The drawing under review shows one solid part. Ordinate dimensions are in mm from its lowest x, y, z. A direction names the side the tool comes from. Give positions to 0.01 mm unless a question says otherwise; leave off trailing zeros. Order: outer loops, then holes, each group sorted by start corner. A loop starts at its lowest first (then second) coordinate and runs counter-clockwise, first axis right, second up. Notation, with made-up numbers: (53.25, 34.5) - (96.25, 34.5) arc R27 ccw to (96.25, 51.5) - close; hole circle Ø8 at (2.5, 31). An arc over 180 degrees is marked (long way). Use CSV: the item, a comma, the result in double quotes.
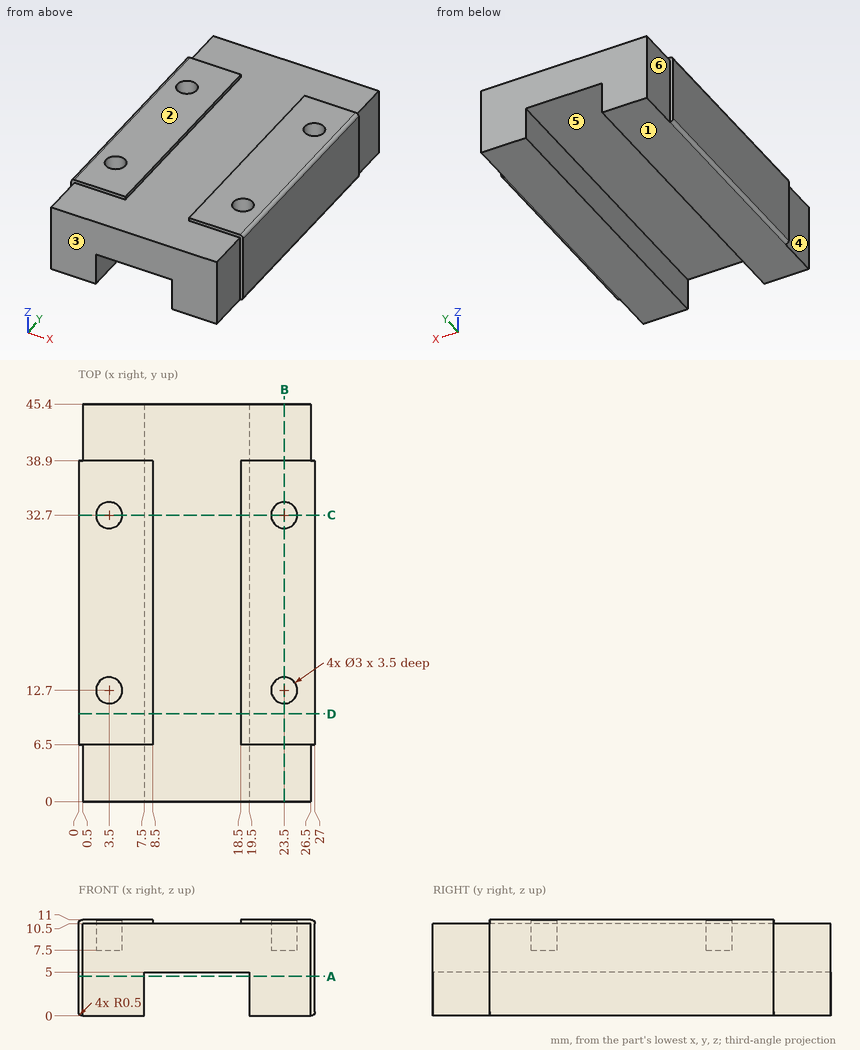
Item 1: Take a section at B-B, the plane x = 23.5. Give the boundary of the cut face in (y, z).
Results list:
outline,"(0, 0) - (45.4, 0) - (45.4, 10.5) - (38.9, 10.5) - (38.9, 11) - (34.2, 11) - (34.2, 7.5) - (31.2, 7.5) - (31.2, 11) - (14.2, 11) - (14.2, 7.5) - (11.2, 7.5) - (11.2, 11) - (6.5, 11) - (6.5, 10.5) - (0, 10.5) - close"
Item 2: Take a section at A-A, the plane z = 4.5. Give the boundary of the cut face in (x, y).
Results list:
outline,"(0, 6.5) - (0.5, 6.5) - (0.5, 0) - (7.5, 0) - (7.5, 45.4) - (0.5, 45.4) - (0.5, 38.9) - (0, 38.9) - close; (19.5, 0) - (26.5, 0) - (26.5, 6.5) - (27, 6.5) - (27, 38.9) - (26.5, 38.9) - (26.5, 45.4) - (19.5, 45.4) - close"
Item 3: Take a section at D-D, the plane y = 10. Give the boundary of the cut face in (x, z).
Results list:
outline,"(0, 0.5) arc R0.5 ccw to (0.5, 0) - (7.5, 0) - (7.5, 5) - (19.5, 5) - (19.5, 0) - (26.5, 0) arc R0.5 ccw to (27, 0.5) - (27, 10.5) arc R0.5 ccw to (26.5, 11) - (18.5, 11) - (18.5, 10.5) - (8.5, 10.5) - (8.5, 11) - (0.5, 11) arc R0.5 ccw to (0, 10.5) - close"
Item 4: Take a section at C-C, the plane y = 32.7. Give the boundary of the cut face in (x, z).
Results list:
outline,"(0, 0.5) arc R0.5 ccw to (0.5, 0) - (7.5, 0) - (7.5, 5) - (19.5, 5) - (19.5, 0) - (26.5, 0) arc R0.5 ccw to (27, 0.5) - (27, 10.5) arc R0.5 ccw to (26.5, 11) - (25, 11) - (25, 7.5) - (22, 7.5) - (22, 11) - (18.5, 11) - (18.5, 10.5) - (8.5, 10.5) - (8.5, 11) - (5, 11) - (5, 7.5) - (2, 7.5) - (2, 11) - (0.5, 11) arc R0.5 ccw to (0, 10.5) - close"
Item 5: Tool access review of the marked faces 4, 5 and 6: name each direction out of +Z, -Z, +X, -X, +Y, -Y from which nothing blocks a thin tool from reaching the whole face with its end or side.
Results list:
face 4,"+Z, -Z, -X, -Y"
face 5,"-Z, +Y, -Y"
face 6,"+Z, -Z, -X, +Y"
Item 6: Wall thickness on L1, parallel to X at y = 12.7, z = 8.9; L2, parallel to Y at x = 3.5, z = 9.15; L3, parallel to X at y = 25.5, z = 3.5: over which ranges is each line inside the solid? List them lowest first.
Results list:
L1,"x = 0 to 2, 5 to 22, 25 to 27"
L2,"y = 0 to 11.2, 14.2 to 31.2, 34.2 to 45.4"
L3,"x = 0 to 7.5, 19.5 to 27"
Item 7: Mouldability with a two-part tool opening along Z and no side actions: class the marked faces 1, 2 and 3 as pulls with the +Z half, pulls with the -Z half, needs draft (parallel to the pull), parting line crosses it, or undercut.
Results list:
face 1,"pulls with the -Z half"
face 2,"pulls with the +Z half"
face 3,"needs draft"
Item 8: Clearance check with flat-ended pins moving along their axes: pin 1 (3.5 mm diameter, centred on x = 23.5, y = 32.7, fed in from +Z); pin 2 (2 mm diameter, centred on y = 43.5, z = 3.5, fed in from -X); pin 3 (0.9 mm diameter, centred on x = 24, y = 12.5, fed in from +Z). State where each tip first meets the part, or that it passes through.
Results list:
pin 1,"stops at z = 11"
pin 2,"stops at x = 0.5"
pin 3,"stops at z = 7.5"
